from build123d import *

# Parameters (mm, degrees)
SKETCH1_W                        = 25
SKETCH1_H                        = 7
BOSS_EXTRUDE1_DEPTH              = 65
SKETCH2_W                        = 11
SKETCH2_H                        = 8
CUT_EXTRUDE1_DEPTH               = 67.560123197
CHAMFER1_SIZE                    = 1
CBORE_FOR_M2_5_SHCS2_D           = 2.9
CBORE_FOR_M2_5_SHCS2_CBORE_D     = 5.5
CBORE_FOR_M2_5_SHCS2_CBORE_DEPTH = 2.5
FILLET1_R                        = 2
FILLET2_R                        = 2
CHAMFER2_SIZE                    = 1


with BuildPart() as part:
    # Sketch1 → Boss-Extrude1 (new body)
    with BuildSketch(Plane.XY):
        Rectangle(SKETCH1_W, SKETCH1_H)
    extrude(amount=BOSS_EXTRUDE1_DEPTH)

    # Sketch2 → Cut-Extrude1 (cut, through all)
    with BuildSketch(Plane(origin=(0, 3.5, 0), x_dir=(1, 0, 0), z_dir=(0, 1, 0))):
        with Locations((0, -61)):
            Rectangle(SKETCH2_W, SKETCH2_H)
    extrude(amount=-CUT_EXTRUDE1_DEPTH, mode=Mode.SUBTRACT)

    # Chamfer1
    chamfer1_edges = [part.edges().sort_by_distance(p)[0] for p in [
        (-5.5, 0, 57),
        (5.5, 0, 57),
    ]]
    chamfer(chamfer1_edges, length=CHAMFER1_SIZE)

    # CBORE for M2.5 SHCS2 (through all)
    with Locations(Plane(origin=(12.5, -6.575007997, 116.706532938), x_dir=(0, 0, -1), z_dir=(1, 0, 0))):
        with Locations((55.706532938, 6.575007997)):
            CounterBoreHole(CBORE_FOR_M2_5_SHCS2_D / 2, CBORE_FOR_M2_5_SHCS2_CBORE_D / 2, CBORE_FOR_M2_5_SHCS2_CBORE_DEPTH)

    # Fillet1
    # the kernel refuses this fillet: 2 mm, written as the material it takes off along each edge
    with BuildSketch(Plane(origin=(12.5, -3.5, -5), x_dir=(-1, 0, 0), z_dir=(0, 0, 1)), Plane(origin=(12.5, 3.5, -5), x_dir=(0, -1, 0), z_dir=(0, 0, 1))) as fillet1_piece_1:
        with BuildLine():
            CenterArc((FILLET1_R, -FILLET1_R), FILLET1_R, 90, 90)
            Line((0, -FILLET1_R), (0, 0))
            Line((0, 0), (FILLET1_R, 0))
        make_face()
    extrude(amount=75, mode=Mode.SUBTRACT)
    with BuildSketch(Plane(origin=(-12.5, -3.5, -5), x_dir=(1, 0, 0), z_dir=(0, 0, 1)), Plane(origin=(-12.5, 3.5, -5), x_dir=(0, -1, 0), z_dir=(0, 0, 1))) as fillet1_piece_2:
        with BuildLine():
            CenterArc((FILLET1_R, FILLET1_R), FILLET1_R, 180, 90)
            Line((0, FILLET1_R), (0, 0))
            Line((0, 0), (FILLET1_R, 0))
        make_face()
    extrude(amount=75, mode=Mode.SUBTRACT)

    # Fillet2
    fillet2_edges = [part.edges().sort_by_distance(p)[0] for p in [
        (-12.5, 0, 0),
        (12.5, 0, 0),
        (0, -3.5, 0),
        (0, 3.5, 0),
        (11.914213562, -2.914213562, 0),
        (-11.914213562, -2.914213562, 0),
        (11.914213562, 2.914213562, 0),
        (-11.914213562, 2.914213562, 0),
    ]]
    fillet(fillet2_edges, radius=FILLET2_R)

    # Chamfer2
    chamfer2_edges = [part.edges().sort_by_distance(p)[0] for p in [
        (-5.5, 0, 65),
        (5.5, 0, 65),
    ]]
    chamfer(chamfer2_edges, length=CHAMFER2_SIZE)


solid = part.part
Geometry check sheet. Reference: the model listing, model coordinates, mm. A direction names the side the tool comes from. Coordinates: 2 decimals unless noted, no trailing zeros. Order: outer loops, then holes, each group sorted by start corner. A loop starts at its lowest first (then second) coordinate and runs counter-clockwise, first axis right, second up. Notation, with made-up numbers: (10.5, 55) - (51.5, 55) arc R11 ccw to (51.5, 64) - close; hole circle Ø3 at (13, -2.5). An arc over 180 degrees is marked (long way). Answer in a Markdown table with one row per item. Add a question column.
1) Material ranges on line 1 along Y through (x, z) = (6.9, 61); line 2 along Y through (x, z) = (10.5, 61); line 3 along Z through (x, y) = (10.65, 0), recorded low to high. Write a range as [from, to].
2) Cross-section at C-C, the plane x = 2.5. Record the cut outline in (y, z), then the cut area to 3 significant figures.
3) Release check for a two-part mould opening along Z. For faces 1 (the flat face through (12.5, 0, 30)), 2 (the cylindrical face through (7.72, 0.06, 59.55)), 3 (the flat face through (-10, 0, 65)), 4 (the flat face through (10, -1.2, 59.8)) record: +Z half, -Z half, draft (parallel to the pull), parting line (faces both ways), or undercut.
4) Set-up check for faces 5 (the flat face through (-12.5, 0, 26)), 6 (the flat face through (5.5, 0.8, 62.4)): record each of +Z, -Z, +X, -X, +Y, -Y from which the full face is reachable in a straight line by a thin tool's end or side.
5) Cross-section at B-B, the plane z = 61. Record the cut outline in (x, y), then the cut area to 3 significant figures.
6) Cross-section at A-A, the plane y = 0. Record the cut outline in (x, z), then the cut area to 3 significant figures.
7) Gauge pin test, flat ends, axial feed: P1, Ø3.5, axis at x = 2, y = 0, coming from the +Z side; P2, Ø3.5, axis at y = 0, z = 61, coming from the +X side. Record the tip position at first contact, or that the pin passes through.
Check result:
| question | item | result |
|---|---|---|
| 1 | line 1 | y = [-3.5, -1.45], [1.45, 3.5] |
| 1 | line 2 | y = [-3.5, -2.75], [2.75, 3.5] |
| 1 | line 3 | z = [0.01, 58.25], [63.75, 65] |
| 2 | outline | (-3.5, 2) arc R2 ccw to (-1.5, 0) - (1.5, 0) arc R2 ccw to (3.5, 2) - (3.5, 57) - (-3.5, 57) - close |
| 2 | area | 397 mm² |
| 3 | face 1 | draft |
| 3 | face 2 | undercut |
| 3 | face 3 | +Z half |
| 3 | face 4 | undercut |
| 4 | face 5 | +Z, -Z, -X, +Y, -Y |
| 4 | face 6 | +Z, +Y, -Y |
| 5 | outline | (-12.5, -1.5) arc R2 ccw to (-10.5, -3.5) - (-5.5, -3.5) - (-5.5, -1.45) - (-12.5, -1.45) - close; (-12.5, 1.45) - (-5.5, 1.45) - (-5.5, 3.5) - (-10.5, 3.5) arc R2 ccw to (-12.5, 1.5) - close; (5.5, -3.5) - (10.5, -3.5) arc R2 ccw to (12.06, -2.75) - (10, -2.75) - (10, -1.45) - (5.5, -1.45) - close; (5.5, 1.45) - (10, 1.45) - (10, 2.75) - (12.06, 2.75) arc R2 ccw to (10.5, 3.5) - (5.5, 3.5) - close |
| 5 | area | 47.8 mm² |
| 6 | outline | (-12.5, 2) arc R2 ccw to (-10.5, 0) - (10.5, 0) arc R2 ccw to (12.5, 2) - (12.5, 58.25) - (10, 58.25) - (10, 59.55) - (5.5, 59.55) - (5.5, 58) - (4.5, 57) - (-4.5, 57) - (-5.5, 58) - (-5.5, 59.55) - (-12.5, 59.55) - close; (-12.5, 62.45) - (-5.5, 62.45) - (-5.5, 64) - (-6.5, 65) - (-12.5, 65) - close; (5.5, 62.45) - (10, 62.45) - (10, 63.75) - (12.5, 63.75) - (12.5, 65) - (6.5, 65) - (5.5, 64) - close |
| 6 | area | 1,490 mm² |
| 7 | P1 | stops at z = 57 |
| 7 | P2 | stops at x = 10 |
